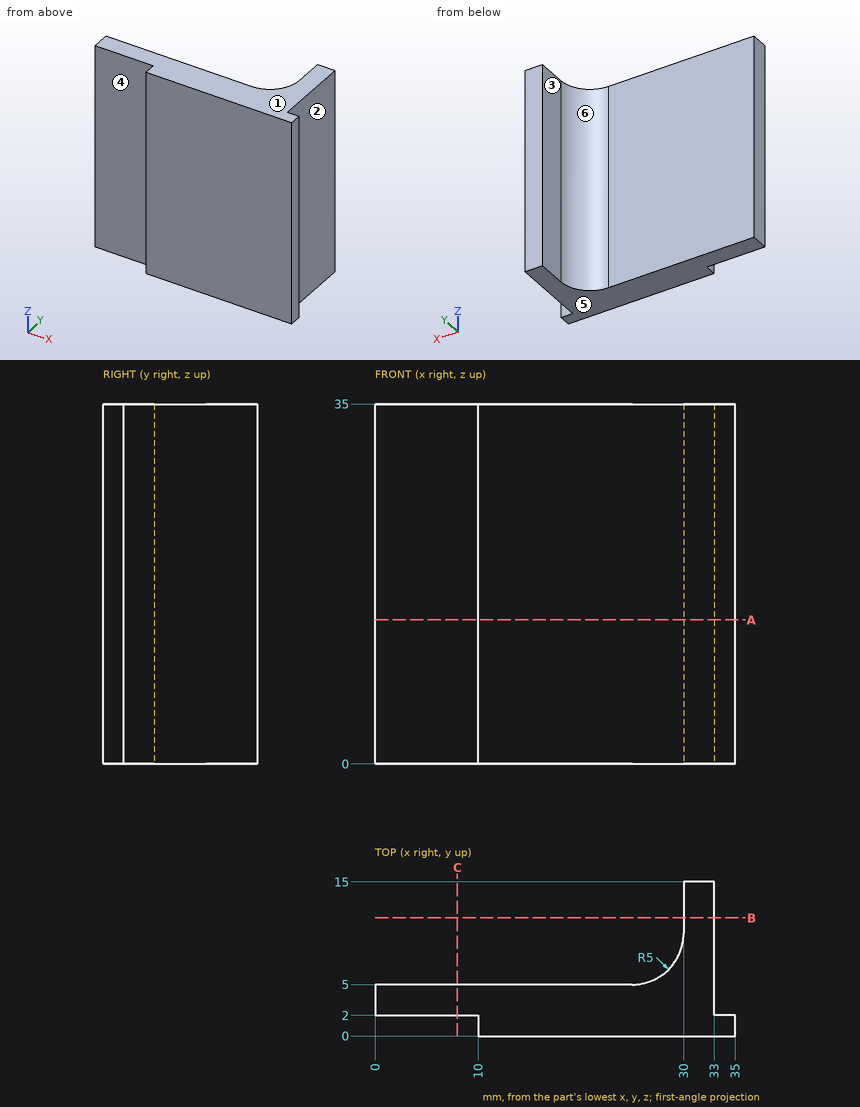
Geometry check sheet. Reference: drawing and pictorial views, mm from the part's lowest x, y, z. A direction names the side the tool comes from. Round coordinates to 2 decimals unless told otherwise and drop trailing zeros. Loops run counter-clockwise (first coordinate to the right, second up) from the corner with the lowest first, then second, coordinate; pieces in that order, holes last.
1. Sectioned sample at A-A on z = 14. Record the boundary of the cut face in (x, y), and give its area (3 significant figures).
2. Sectioned sample at B-B on y = 11.5. Record the boundary of the cut face in (x, z).
3. Set-up check for the marked faces 1, 2 and 3: record each of +Z, -Z, +X, -X, +Y, -Y from which the full face is reachable in a straight line by a thin tool's end or side.
4. Scan lines: probe 1 along Y at (x, z) = (9.5, 26); probe 2 along Y at (x, z) = (18, 25); probe 3 along X at (y, z) = (14.75, 14). Record each from-to range of solid material in increasing order.
5. Sectioned sample at C-C on x = 8. Record the boundary of the cut face in (y, z).
6. Gauge pin test, flat ends, axial feed: pin 1 Ø5 at (x, z) = (6, 17) entering from -Y; pin 2 Ø2 at (x, z) = (7, 28) entering from +Y; pin 3 Ø1 at (x, z) = (34, 15.5) entering from +Y; pin 4 Ø2 at (x, y) = (15, 7.5) entering from -Z. Record the tip position at first contact, or that the pin passes through.
7. Mould release check, pull along Y, two halves, no side actions. Record for the marked faces 4, 5 and 6: released by +Y, released by -Y, zero draft, split by the parting line, or undercut.
Recorded:
1. outline: (0, 2) - (10, 2) - (10, 0) - (35, 0) - (35, 2) - (33, 2) - (33, 15) - (30, 15) - (30, 10) arc R5 cw to (25, 5) - (0, 5) - close
1. area: 184 mm2
2. outline: (30, 0) - (33, 0) - (33, 35) - (30, 35) - close
3. face 1: +Z, +X, -X, +Y, -Y
3. face 2: +Z, -Z, +X, +Y
3. face 3: +Z, -Z, -X, +Y
4. probe 1: y = 2 to 5
4. probe 2: y = 0 to 5
4. probe 3: x = 30 to 33
5. outline: (2, 0) - (5, 0) - (5, 35) - (2, 35) - close
6. pin 1: stops at y = 2
6. pin 2: stops at y = 5
6. pin 3: stops at y = 2
6. pin 4: passes through
7. face 4: released by -Y
7. face 5: zero draft
7. face 6: released by +Y
